Geometry: final body of the model. Coordinates: model frame, mm. Face numbers are marked on the shaded views. A direction names the side the tool comes from. Give positions to 0.01 mm unless a question says otherwise; leave off trailing zeros. Write each loop counter-clockwise with the first axis right and the second up, starting at its lowest first coordinate (ties: lowest second). Pieces come first, ordered by that corner, then holes.
Q1. Reachability of the marked faces 1, 2 and 3 from +Z, -Z, +X, -X, +Y, -Y: full face, straight path, thin tool, end or side. Return the list, or none.
Q2. Pin query (flat end, axial travel): pin 1 Ø4 at (x, y) = (54.5, -4) entering from -Z. Return the tip coordinate at first contact, or that it passes through.
Q3. Line query: line 1 (X direction, y = -5.25, z = 3.25); line 2 (Y direction, x = 38, z = 0.5); line 3 (Z direction, x = 20, y = -1). Output: solid intervals per line, ascending.
Q4. Section C-C (x = 24). Return the cut outline in (y, z).
Q5. Section A-A (z = 0). Return the cut outline in (x, y) (3 decimals), plus the area to 3 significant figures.
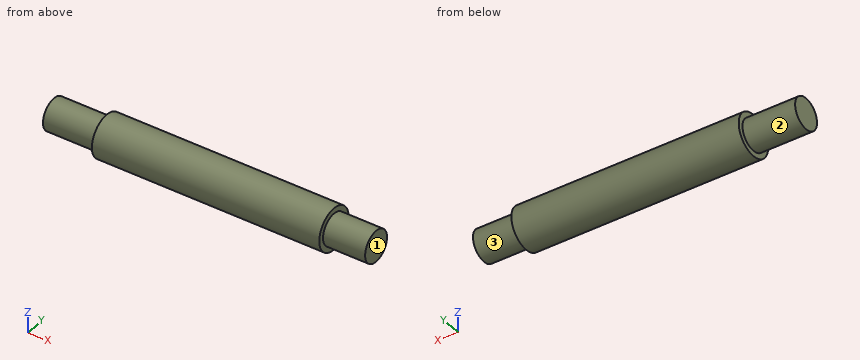
from build123d import *

# Parameters (mm, degrees)
F0_R     = 6.3246
F1_DEPTH = 68.58
F2_R     = 4.7117
F3_DEPTH = 12.7
F4_R     = 4.7117
F5_DEPTH = 15.875


with BuildPart() as f1:
    # F0 (on Right) → F1 (new body)
    with BuildSketch(Plane.YZ):
        Circle(F0_R)
    extrude(amount=F1_DEPTH)

    # F2 (on face) → F3 (join)
    with BuildSketch(Plane.YZ.offset(68.58)):
        Circle(F2_R)
    extrude(amount=F3_DEPTH)

    # F4 (on face) → F5 (join)
    with BuildSketch(Plane(origin=(0, 0, 0), x_dir=(0, -1, 0), z_dir=(-1, 0, 0))):
        Circle(F4_R)
    extrude(amount=F5_DEPTH)


solid = f1.part
Computed:
1. face 1: +Z, -Z, +X, +Y, -Y
1. face 2: -X
1. face 3: +X
2. pin 1: stops at z = -6
3. line 1: x = 0 to 68.58
3. line 2: y = -6.3 to 6.3
3. line 3: z = -6.25 to 6.25
4. outline: circle Ø12.65 at (0, 0)
5. outline: (-15.875, -4.712) - (0, -4.712) - (0, -6.325) - (68.58, -6.325) - (68.58, -4.712) - (81.28, -4.712) - (81.28, 4.712) - (68.58, 4.712) - (68.58, 6.325) - (0, 6.325) - (0, 4.712) - (-15.875, 4.712) - close
5. area: 1,140 mm2
